```python
from build123d import *

# Parameters (mm, degrees)
F3_R     = 0.508
F6_R     = 0.5207
F7_DEPTH = 9.7165


# Not quite as in the source:
# - a fillet or chamfer that OpenCascade refuses, or shapes differently, is made with other operations: its cross-section is extruded or revolved along the edge and cut away or added


with BuildPart() as f1:
    # F0 (on Front) → F1 (revolve)
    with BuildSketch(Plane.XZ):
        Polygon((0, 4.6355), (0, 0), (38.1, 0), (38.1, 1.5875), (1.905, 1.5875), (1.905, 3.2385), (0.508, 4.6355), align=None)
    revolve(axis=Axis((19.05, 0, 0), (1, 0, 0)))

    # F2: fillet of radius 2.032 on 1 edges, made by hand

    # F2_s1 → F2_t2 (revolve)
    with BuildSketch(Plane.XZ):
        with BuildLine():
            ThreePointArc((1.905, 3.2385), (2.6058107165, 2.0537388432), (3.900961673, 1.5875))
            Line((3.900961673, 1.5875), (3.900961673, 1.54686))
            Line((3.900961673, 1.54686), (1.905, 1.54686))
            Line((1.905, 1.54686), (1.86436, 1.5875))
            ThreePointArc((1.86436, 1.5875), (1.86436, 2.413), (1.8650807665, 3.23088))
            Line((1.8650807665, 3.23088), (1.905, 3.2385))
        make_face()
    revolve(axis=Axis((1.905, 0, 0), (1, 0, 0)))

    # F3
    f3_edges = [f1.edges().sort_by_distance(p)[0] for p in [
        (38.1, 0, -1.5875),
    ]]
    fillet(f3_edges, radius=F3_R)

    # F6 (on offset) → F7 (cut, through all)
    with BuildSketch(Plane.XZ.offset(5.08)):
        with Locations((36.195, 0)):
            Circle(F6_R)
    extrude(amount=-F7_DEPTH, mode=Mode.SUBTRACT)


solid = f1.part
```
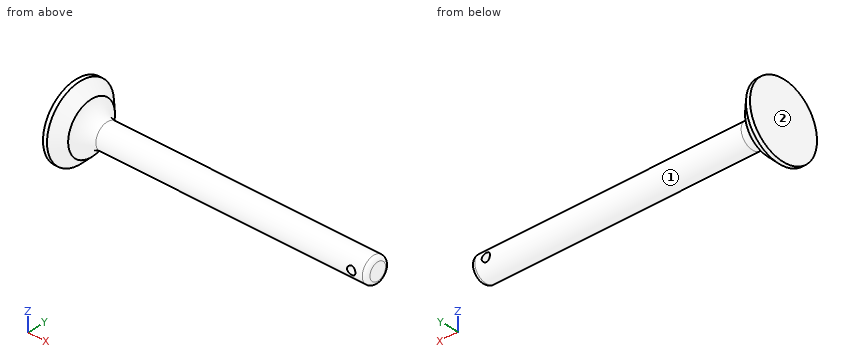
Geometry check sheet. Reference: the model listing, model coordinates, mm. Face numbers are marked on the shaded views. A direction names the side the tool comes from. Coordinates: 2 decimals unless noted, no trailing zeros. Order: outer loops, then holes, each group sorted by start corner. A loop starts at its lowest first (then second) coordinate and runs counter-clockwise, first axis right, second up.
Item 1: Depth check by flat-ended pin: pin 1 (3 mm diameter, centred on x = 10.5, z = 0, fed in from +Y); pin 2 (1 mm diameter, centred on x = 11.5, z = 1.5, fed in from +Y); pin 3 (4 mm diameter, centred on x = 31, z = 2.5, fed in from +Y). Enter the tip coordinate at first touch or a pass-through.
Item 2: Tool access check on the marked faces 1 and 2. Record the directions out of +Z, -Z, +X, -X, +Y, -Y that give a thin tool (end or side, any length) a straight path to the whole face; none if there is none.
Item 3: Section check C-C (x = 27). Enter the section's corners in (y, z) (1 decimal).
Item 4: Section check A-A (y = 0). Enter the section's corners in (x, z) (1 decimal).
Item 5: Scan lines: line 1 along X through (y, z) = (0.5, 0); line 2 along Y through (x, z) = (29, 0); line 3 along Z through (x, y) = (28.5, -0.5). Record each from-to range of solid material in increasing order.
Item 6: Section check B-B (z = 0). Enter the section's corners in (x, y) (1 decimal), plus the area to 3 significant figures.
Check sheet entries:
1. pin 1: stops at y = 1.59
1. pin 2: stops at y = 1.23
1. pin 3: stops at y = 1.51
2. face 1: +X
2. face 2: +Z, -Z, -X, +Y, -Y
3. outline: circle Ø3.2 at (0, 0)
4. outline: (0, -4.6) - (0.5, -4.6) - (1.9, -3.2) arc R2 cw to (3.9, -1.6) - (37.6, -1.6) arc R0.5 ccw to (38.1, -1.1) - (38.1, 1.1) arc R0.5 ccw to (37.6, 1.6) - (3.9, 1.6) arc R2 cw to (1.9, 3.2) - (0.5, 4.6) - (0, 4.6) - close; hole circle Ø1 at (36.2, 0)
5. line 1: x = 0 to 35.67, 36.72 to 38.1
5. line 2: y = -1.59 to 1.59
5. line 3: z = -1.51 to 1.51
6. outline: (0, -4.6) - (0.5, -4.6) - (1.9, -3.2) arc R2 cw to (3.9, -1.6) - (35.7, -1.6) - (35.7, 1.6) - (3.9, 1.6) arc R2 cw to (1.9, 3.2) - (0.5, 4.6) - (0, 4.6) - close; (36.7, -1.6) - (37.6, -1.6) arc R0.5 ccw to (38.1, -1.1) - (38.1, 1.1) arc R0.5 ccw to (37.6, 1.6) - (36.7, 1.6) - close
6. area: 129 mm2
